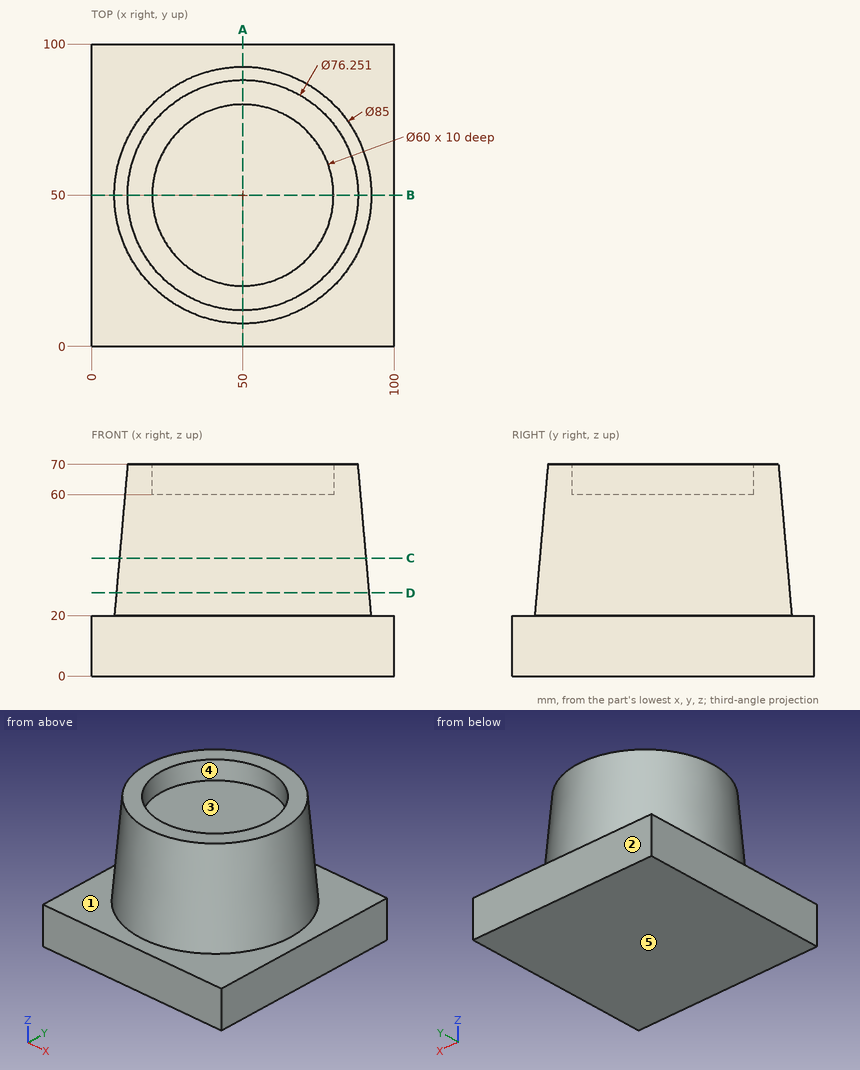
For this review, use the dimensioned drawing (mm, ordinates from the lowest corner) and the shaded views. A direction names the side the tool comes from. Coordinates: 2 decimals unless noted, no trailing zeros. Order: outer loops, then holes, each group sorted by start corner. A loop starts at its lowest first (then second) coordinate and runs counter-clockwise, first axis right, second up. Notation, with made-up numbers: (23, -15) - (63, -15) arc R24 cw to (63, -5) - close; hole circle Ø9 at (71.25, 28.5). An arc over 180 degrees is marked (long way). Answer as a JSON object with one key per item and string values. Group by question number.
1. We need section C-C on z = 39. State the section outline as (x, y) points.
2. For the marked faces 4 and 5, list the 3-axis set-ups (+Z, -Z, +X, -X, +Y, -Y) from which the entire face can be reached by the end or side of a thin tool; tool diameter is ignored.
3. The part is to be moulded in two halves that separate along Y. For the marked faces 1, 2 and 3, say which applies: pulls with the +Y half, pulls with the -Y half, needs draft (parallel to the pull), parting line crosses it, or undercut.
4. We need section A-A on x = 50. State the section outline as (y, z) points, then the cut area to 3 significant figures.
5. Clearance check with flat-ended pins moving along their axes: P1, Ø3, axis at x = 60.5, z = 22, coming from the -Y side; P2, Ø1.5, axis at x = 78.5, y = 50, coming from the +Z side. State where each tip first meets the part, or that it passes through.
6. We need section D-D on z = 27.5. State the section outline as (x, y) points.
7. For probe 1 along Z at (x, y) = (48, 70); probe 2 along Z at (x, y) = (90, 9); probe 3 along Y at (x, z) = (50, 64.75) (3 decimals), list the stretches that pass through material, from the lowest coordinate up.
Final values:
{
 "1": {"outline": "circle Ø81.68 at (50, 50)"},
 "2": {"face 4": "+Z", "face 5": "-Z, +X, -X, +Y, -Y"},
 "3": {"face 1": "needs draft", "face 2": "pulls with the +Y half", "face 3": "undercut"},
 "4": {"outline": "(0, 0) - (100, 0) - (100, 20) - (92.5, 20) - (88.13, 70) - (80, 70) - (80, 60) - (20, 60) - (20, 70) - (11.87, 70) - (7.5, 20) - (0, 20) - close", "area": "5,430 mm²"},
 "5": {"P1": "y = 8.62", "P2": "z = 60"},
 "6": {"outline": "circle Ø83.69 at (50, 50)"},
 "7": {"probe 1": "0 to 60", "probe 2": "0 to 20", "probe 3": "11.415 to 20, 80 to 88.585"}
}
